The model under review builds one solid part; all positions refer to its coordinate system, in mm. Coordinates: 2 decimals unless noted, no trailing zeros. Loops run counter-clockwise (first coordinate to the right, second up) from the corner with the lowest first, then second, coordinate; pieces in that order, holes last. Notation, with made-up numbers: M -6.75,74.25 L 21.25,74.25 A9 ccw 21.25,83.25 Z; hole C -1,21.5 d1. An arc over 180 degrees is marked long. Use CSV: the item, a comma, the result in double quotes. Start each with the question number.
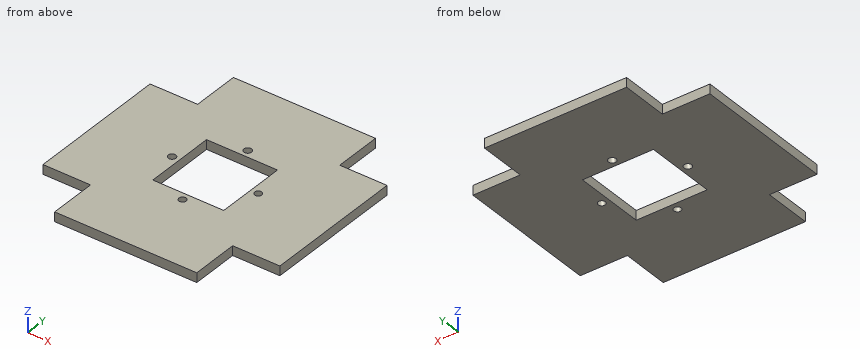
from build123d import *

# Parameters (mm, degrees)
SKETCH2_R           = 2.08028948
SKETCH2_R_2         = 1.930605223
SKETCH2_R_3         = 1.931643465
SKETCH2_R_4         = 2.051960052
SKETCH2_W           = 38.050309674
SKETCH2_H           = 38.166973502
BOSS_EXTRUDE1_DEPTH = 5.08


with BuildPart() as part:
    # Sketch2 → Boss-Extrude1 (new body)
    with BuildSketch(Plane.XY):
        Polygon((49.372044396, 30.512685118), (-26.811291054, 30.512685118), (-26.811291054, 5.122215891), (-52.307460203, 5.122215891), (-52.307460203, -70.962795052), (-26.811291054, -70.962795052), (-26.811291054, -96.487314882), (49.372044396, -96.487314882), (49.372044396, -70.962795052), (74.692539797, -70.962795052), (74.692539797, 5.122215891), (49.372044396, 5.122215891), align=None)
        with Locations((11.280376671, -9.772802829)):
            Circle(SKETCH2_R, mode=Mode.SUBTRACT)
        with Locations((34.369531508, -32.92028958)):
            Circle(SKETCH2_R_2, mode=Mode.SUBTRACT)
        with Locations((11.280376671, -56.067776331)):
            Circle(SKETCH2_R_3, mode=Mode.SUBTRACT)
        with Locations((-11.808778166, -32.92028958)):
            Circle(SKETCH2_R_4, mode=Mode.SUBTRACT)
        with Locations((11.280376671, -32.92028958)):
            Rectangle(SKETCH2_W, SKETCH2_H, mode=Mode.SUBTRACT)
    extrude(amount=BOSS_EXTRUDE1_DEPTH)


solid = part.part
1. Insertion check: pin 1 Ø2.5 at (x, z) = (56, 2.5) entering from +Y; pin 2 Ø2.5 at (x, z) = (-42, 3) entering from -Y. Each pin has a flat end and moves straight along its axis. Give the tip position at first contact, or say it passes through.
2. Add section A-A (x = 6). Write out the cut boundary in (y, z), plus the area to 3 significant figures.
3. To check wall thickness, follow line 1 along X through (y, z) = (-45, 1.6); line 2 along X through (y, z) = (-33.5, 4.25); line 3 along Y through (x, z) = (-12.5, 2.4). State the ranges of each line that lie inside material, in increasing order.
4. Add section B-B (y = -20.5). Write out the cut boundary in (x, z).
5. Add section C-C (z = 2.9). Write out the cut boundary in (x, y), plus the area to 3 significant figures.
6. Add section D-D (y = -87). Write out the cut boundary in (x, z), plus the area to 3 significant figures.
Solved:
1,pin 1,"stops at y = 5.12"
1,pin 2,"stops at y = -70.96"
2,outline,"M -96.49,0 L -52,0 L -52,5.08 L -96.49,5.08 Z; M -13.84,0 L 30.51,0 L 30.51,5.08 L -13.84,5.08 Z"
2,area,"451 mm^2"
3,line 1,"x = -52.31 to -7.74, 30.31 to 74.69"
3,line 2,"x = -52.31 to -13.78, -9.84 to -7.74, 30.31 to 32.53, 36.21 to 74.69"
3,line 3,"y = -96.49 to -34.85, -30.99 to 30.51"
4,outline,"M -52.31,0 L -7.74,0 L -7.74,5.08 L -52.31,5.08 Z; M 30.31,0 L 74.69,0 L 74.69,5.08 L 30.31,5.08 Z"
5,outline,"M -52.31,-70.96 L -26.81,-70.96 L -26.81,-96.49 L 49.37,-96.49 L 49.37,-70.96 L 74.69,-70.96 L 74.69,5.12 L 49.37,5.12 L 49.37,30.51 L -26.81,30.51 L -26.81,5.12 L -52.31,5.12 Z; hole C -11.81,-32.92 d4.1; hole M -7.74,-52 L 30.31,-52 L 30.31,-13.84 L -7.74,-13.84 Z; hole C 11.28,-9.77 d4.16; hole C 11.28,-56.07 d3.86; hole C 34.37,-32.92 d3.86"
5,area,"12,000 mm^2"
6,outline,"M -26.81,0 L 49.37,0 L 49.37,5.08 L -26.81,5.08 Z"
6,area,"387 mm^2"
